from build123d import *

# Parameters (mm, degrees)
SKETCH_1_W          = 100
SKETCH_1_H          = 100
EXTRUDE_1_DEPTH     = 6
SKETCH_2_W          = 7
SKETCH_2_H          = 6
EXTRUDE_2_DEPTH     = 6
CUT_EXTRUDE_1_DEPTH = 7


with BuildPart() as part:
    # Эскиз1 → Бобышка-Вытянуть1 (new body)
    with BuildSketch(Plane.XY):
        Rectangle(SKETCH_1_W, SKETCH_1_H)
    extrude(amount=EXTRUDE_1_DEPTH)

    # Эскиз2 → Бобышка-Вытянуть2 (add)
    with BuildSketch(Plane.XY.offset(6)):
        with Locations((-9.531849908, 53)):
            Rectangle(SKETCH_2_W, SKETCH_2_H)
        with Locations((9.531849908, 53)):
            Rectangle(SKETCH_2_W, SKETCH_2_H)
    extrude(amount=-EXTRUDE_2_DEPTH)

    # Эскиз3 → Вырез-Вытянуть1 (cut, through all)
    with BuildSketch(Plane.XY.offset(6)):
        Polygon((-2.1, 45), (-3.6, 45), (-3.6, 42.6), (-2.1, 42.6), (-2.1, 39), (2.1, 39), (2.1, 42.6), (3.6, 42.6), (3.6, 45), (2.1, 45), (2.1, 50), (-2.1, 50), align=None)
    extrude(amount=-CUT_EXTRUDE_1_DEPTH, mode=Mode.SUBTRACT)


solid = part.part
Could you check a few things on this model? Use its own coordinates, in mm. A direction names the side the tool comes from. Give positions to 0.01 mm unless a question says otherwise; leave off trailing zeros. Loops run counter-clockwise (first coordinate to the right, second up) from the corner with the lowest first, then second, coordinate; pieces in that order, holes last. Notation, with made-up numbers: (-15, -34.5) -> (-9, -34.5) arc R17 cw to (-9, -25.5) -> close; hole circle Ø5 at (13, 87.25). An arc over 180 degrees is marked (long way). Answer as CSV lines item,"result". Start each with the question number.
(1) If we section it at A-A on z = 2.7: Write out the boundary of the cut face in (x, y), then the cut area to 3 significant figures.
(2) Which directions (+Z, -Z, +X, -X, +Y, -Y) give clear straight access to the entire face, cutting with the end or side of a thin tool? Please do faces 1 (the flat face through (4, 50, 3)), 2 (the flat face through (-32, 50, 3)), 3 (the flat face through (-3.6, 44, 3)).
(3) I need wall thicknesses on probe 1 along X at (y, z) = (51, 4.7); probe 2 along X at (y, z) = (44, 4.3); probe 3 along Y at (x, z) = (-2.5, 1.3). Which ranges of each line are inside material? Lowest first, please.
(4) We'd pull the mould along X, two halves only. Please class faces 4 (the flat face through (-4, 50, 3)), 5 (the flat face through (31, 50, 3)), 6 (the flat face through (-50, -1, 3)): released by +X, released by -X, zero draft, split by the parting line, or undercut.
(5) If we section it at B-B on x = -15: Write out the boundary of the cut face in (y, z).
(6) I'm going to push flat-ended pins straight in: pin 1 Ø1.8 at (y, z) = (53, 4) entering from -X; pin 2 Ø2 at (x, z) = (0.5, 3.5) entering from +Y; pin 3 Ø1.6 at (x, z) = (-2.5, 3.5) entering from +Y. Where does each tip first touch, or does it pass through?
Computed:
1,outline,"(-50, -50) -> (50, -50) -> (50, 50) -> (13.03, 50) -> (13.03, 56) -> (6.03, 56) -> (6.03, 50) -> (2.1, 50) -> (2.1, 45) -> (3.6, 45) -> (3.6, 42.6) -> (2.1, 42.6) -> (2.1, 39) -> (-2.1, 39) -> (-2.1, 42.6) -> (-3.6, 42.6) -> (-3.6, 45) -> (-2.1, 45) -> (-2.1, 50) -> (-6.03, 50) -> (-6.03, 56) -> (-13.03, 56) -> (-13.03, 50) -> (-50, 50) -> close"
1,area,"10,000 mm2"
2,face 1,"+Z, -Z, +Y"
2,face 2,"+Z, -Z, -X, +Y"
2,face 3,"+Z, -Z"
3,probe 1,"x = -13.03 to -6.03, 6.03 to 13.03"
3,probe 2,"x = -50 to -3.6, 3.6 to 50"
3,probe 3,"y = -50 to 42.6, 45 to 50"
4,face 4,"undercut"
4,face 5,"zero draft"
4,face 6,"released by -X"
5,outline,"(-50, 0) -> (50, 0) -> (50, 6) -> (-50, 6) -> close"
6,pin 1,"stops at x = -13.03"
6,pin 2,"stops at y = 39"
6,pin 3,"stops at y = 50"
